The drawing under review shows one solid part. Ordinate dimensions are in mm from its lowest x, y, z. Coordinates: 2 decimals unless noted, no trailing zeros. Write each loop counter-clockwise with the first axis right and the second up, starting at its lowest first coordinate (ties: lowest second). Pieces come first, ordered by that corner, then holes. Notation, with made-up numbers: M 70,24 L 115,24 A20 ccw 115,59 Z; hole C 59,69.5 d11. An arc over 180 degrees is marked long. Write each question's results on one line, items separated by ' | '. Start each with the question number.
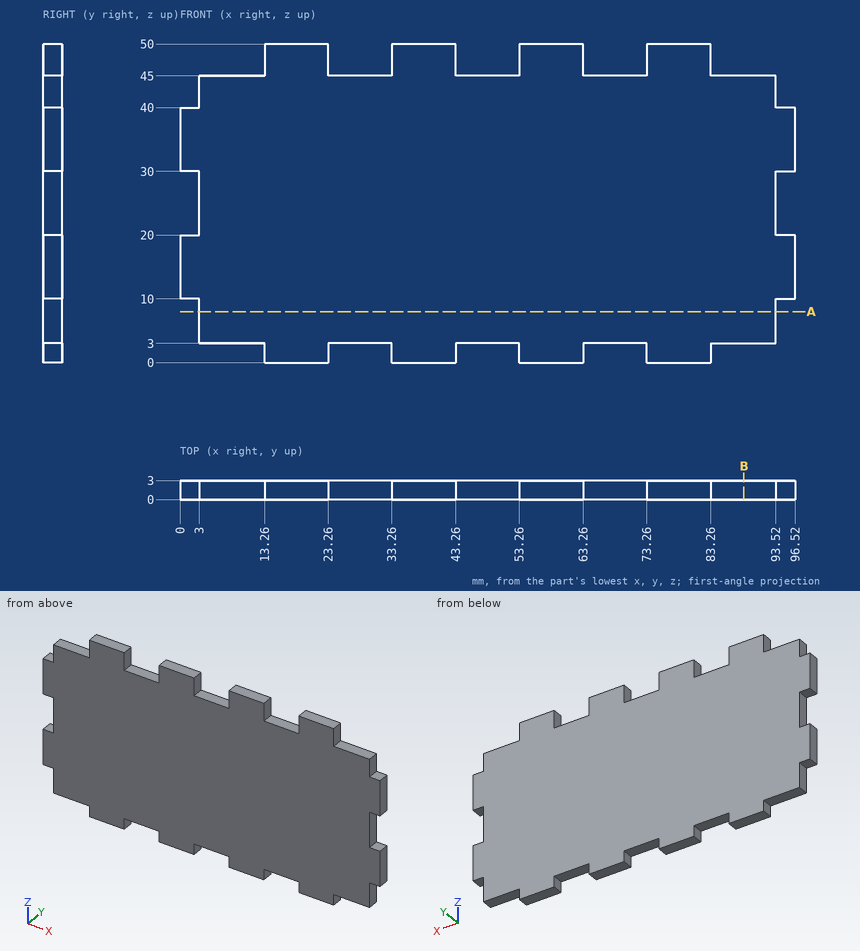
Item 1: We need section B-B on x = 88.5. State the section outline as (y, z) points, then the cut area to 3 significant figures.
Item 2: We need section A-A on z = 8. State the section outline as (x, y) points.
Item 3: Wall thickness on L1, parallel to X at y = 2.4, z = 46; L2, parallel to Z at x = 32.5, y = 2; L3, parallel to X at y = 0.4, z = 23.5: over which ranges is each line inside the solid? List them lowest first.
Item 4: Insertion check: pin 1 Ø0.9 at (x, y) = (9, 1.5) entering from -Z; pin 2 Ø1.5 at (x, y) = (95.5, 2) entering from -Z; pin 3 Ø0.9 at (y, z) = (1, 48.5) entering from -X. Each pin has a flat end and moves straight along its axis. Give the tip position at first contact, or say it passes through.
Answer:
1) outline: M 0,3 L 3,3 L 3,45 L 0,45 Z | area: 126 mm^2
2) outline: M 3,0 L 93.52,0 L 93.52,3 L 3,3 Z
3) L1: x = 13.26 to 23.26, 33.26 to 43.26, 53.26 to 63.26, 73.26 to 83.26 | L2: z = 3 to 45 | L3: x = 3 to 93.52
4) pin 1: stops at z = 3 | pin 2: stops at z = 10 | pin 3: stops at x = 13.26
